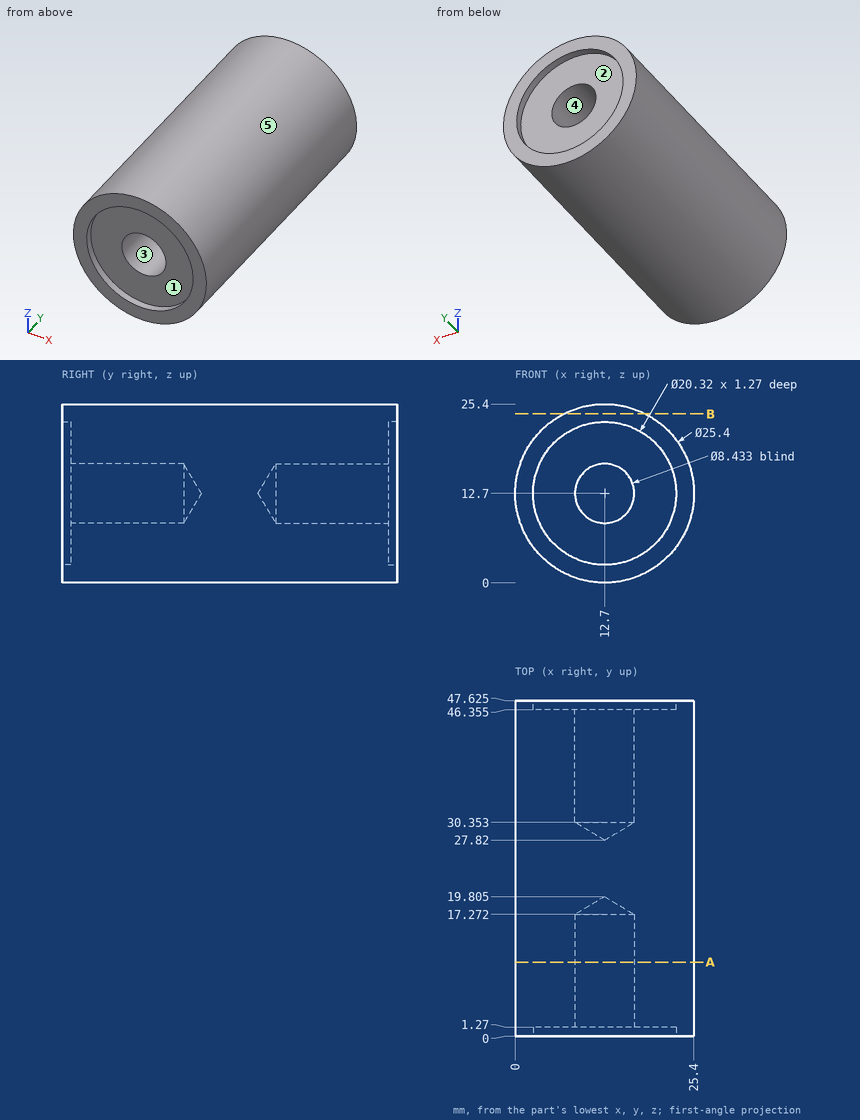
Geometry check sheet. Reference: drawing and pictorial views, mm from the part's lowest x, y, z. A direction names the side the tool comes from. Give positions to 0.01 mm unless a question says otherwise; leave off trailing zeros. Loops run counter-clockwise (first coordinate to the right, second up) from the corner with the lowest first, then second, coordinate; pieces in that order, holes last.
1. Set-up check for the marked faces 1 and 2: record each of +Z, -Z, +X, -X, +Y, -Y from which the full face is reachable in a straight line by a thin tool's end or side.
2. Section check B-B, the plane z = 24. Enter the section's corners in (x, y) (1 decimal).
3. Go/stop test with flat-tipped pins: pin 1 Ø1 at (x, y) = (17, 17) entering from -Z; pin 2 Ø2 at (x, y) = (7, 20.5) entering from -Z; pin 3 Ø13.5 at (x, z) = (12.7, 12.7) entering from -Y; pin 4 Ø12 at (x, y) = (7, 30) entering from +Z. Record where each tip stops, or that it passes through.
4. Mould release check, pull along X, two halves, no side actions. Record for the marked faces 3, 4 and 5: released by +X, released by -X, zero draft, split by the parting line, or undercut.
5. Thickness scan on line 1 (X direction, y = 43.25, z = 12.7); line 2 (X direction, y = 46.95, z = 12.7); line 3 (Z direction, x = 12.5, y = 5). Record the ranges inside material, lowest first.
6. Section check A-A, the plane y = 10.5. Enter the section's corners in (x, z).
Geometry says:
1. face 1: -Y
1. face 2: +Y
2. outline: (6.9, 0) - (18.5, 0) - (18.5, 47.6) - (6.9, 47.6) - close
3. pin 1: stops at z = 0.58
3. pin 2: stops at z = 0.9
3. pin 3: stops at y = 1.27
3. pin 4: stops at z = 25.4
4. face 3: undercut
4. face 4: undercut
4. face 5: split by the parting line
5. line 1: x = 0 to 8.48, 16.92 to 25.4
5. line 2: x = 0 to 2.54, 22.86 to 25.4
5. line 3: z = 0 to 8.49, 16.91 to 25.4
6. outline: circle Ø25.4 at (12.7, 12.7); hole circle Ø8.43 at (12.7, 12.7)
